Verification items for the finished model (mm, model axes). A direction names the side the tool comes from. Give positions to 0.01 mm unless a question says otherwise; leave off trailing zeros. Order: outer loops, then holes, each group sorted by start corner. A loop starts at its lowest first (then second) coordinate and runs counter-clockwise, first axis right, second up. Notation, with made-up numbers: (-37, 52) - (-10, 52) arc R10 ccw to (-10, 70) - close; hole circle Ø10 at (58, 86.5). An arc over 180 degrees is marked (long way). Answer as a JSON object with one key per item and string values.
```python
from build123d import *

# Parameters (mm, degrees)
F0_R     = 12
F1_DEPTH = 19
F3_R     = 12
F3_R_2   = 10
F4_DEPTH = 13
F6_R     = 5
F7_DEPTH = 25
F8_R     = 10.5
F9_DEPTH = 5
F10_SIZE = 3.5


with BuildPart() as f1:
    # F0 (on Front) → F1 (new body)
    with BuildSketch(Plane.XZ):
        Circle(F0_R)
    extrude(amount=-F1_DEPTH)

    # F3 (on offset) → F4 (cut)
    with BuildSketch(Plane.XZ.offset(-10.5)):
        Circle(F3_R)
        Circle(F3_R_2, mode=Mode.SUBTRACT)
    extrude(amount=-F4_DEPTH, mode=Mode.SUBTRACT)

    # F6 (on offset) → F7 (cut)
    with BuildSketch(Plane(origin=(0, 19, 0), x_dir=(1, 0, 0), z_dir=(0, 1, 0))):
        Circle(F6_R)
    extrude(amount=-F7_DEPTH, mode=Mode.SUBTRACT)

    # F8 (on Front) → F9 (cut)
    with BuildSketch(Plane.XZ):
        Circle(F8_R)
    extrude(amount=-F9_DEPTH, mode=Mode.SUBTRACT)

    # F10
    f10_edges = [f1.edges().sort_by_distance(p)[0] for p in [
        (-10, 19, 0),
    ]]
    chamfer(f10_edges, length=F10_SIZE)


solid = f1.part
```
(1) Section check A-A (z = 0). Record the cut outline in (x, y), then the cut area to 3 significant figures.
Computed values:
{"outline": "(-12, 0) - (-10.5, 0) - (-10.5, 5) - (-5, 5) - (-5, 19) - (-6.5, 19) - (-10, 15.5) - (-10, 10.5) - (-12, 10.5) - close; (5, 5) - (10.5, 5) - (10.5, 0) - (12, 0) - (12, 10.5) - (10, 10.5) - (10, 15.5) - (6.5, 19) - (5, 19) - close", "area": "165 mm²"}
(2) Material ranges on line 1 along Z through (x, y) = (0, 3.6); line 2 along Z through (x, y) = (0, 6.75); line 3 along X through (y, z) = (9, 4), recorded low to high. Write a range as [from, to].
Computed values:
{"line 1": "z = [-12, -10.5], [10.5, 12]", "line 2": "z = [-12, -5], [5, 12]", "line 3": "x = [-11.31, -3], [3, 11.31]"}
(3) Access from +Z, -Z, +X, -X, +Y, -Y to the whole of each face (thin tool, end or side, straight path). Record for faces 1 (the flat face through (2, 19, -5)), 2 (the cylindrical face through (10, 2.5, 3.2)).
Computed values:
{"face 1": "+Z, -Z, +X, -X, +Y", "face 2": "-Y"}
(4) Gauge pin test, flat ends, axial feed: pin 1 Ø8 at (y, z) = (10, 2.5) entering from +X; pin 2 Ø3 at (x, z) = (-6, 6) entering from +Y; pin 3 Ø2 at (y, z) = (2, 7.5) entering from -X; pin 4 Ø6 at (y, z) = (6.5, -9.5) entering from +X. Record the tip position at first contact, or that the pin passes through.
Computed values:
{"pin 1": "stops at x = 12", "pin 2": "stops at y = 18.51", "pin 3": "stops at x = -10.09", "pin 4": "stops at x = 10.09"}
(5) Section check D-D (y = 11.5). Record the cut outline in (x, z).
Computed values:
{"outline": "circle Ø20 at (0, 0); hole circle Ø10 at (0, 0)"}
(6) Release check for a two-part mould opening along X. For faces 3 (the flat face through (5, 5, -2)), 4 (the flat face through (-5, 10.5, 9)), 5 (the cylindrical face through (-2.17, 12.96, -9.76)) record: pulls with the +X half, pulls with the -X half, needs draft (parallel to the pull), parting line crosses it, or undercut.
Computed values:
{"face 3": "undercut", "face 4": "needs draft", "face 5": "parting line crosses it"}
(7) Section check B-B (x = 0). Record the cut outline in (y, z), then the cut area to 3 significant figures.
Computed values:
{"outline": "(0, -12) - (10.5, -12) - (10.5, -10) - (15.5, -10) - (19, -6.5) - (19, -5) - (5, -5) - (5, -10.5) - (0, -10.5) - close; (0, 10.5) - (5, 10.5) - (5, 5) - (19, 5) - (19, 6.5) - (15.5, 10) - (10.5, 10) - (10.5, 12) - (0, 12) - close", "area": "165 mm²"}
(8) Section check C-C (y = 9.25). Record the cut outline in (x, z).
Computed values:
{"outline": "circle Ø24 at (0, 0); hole circle Ø10 at (0, 0)"}
